```python
from build123d import *

# Parameters (mm, degrees)
SKETCH_1_R          = 32.5
SKETCH_1_R_2        = 17.5
SKETCH_1_R_3        = 2.5
EXTRUDE_1_DEPTH     = 24
SKETCH_2_R          = 35
SKETCH_2_R_2        = 21.5
CUT_EXTRUDE_2_DEPTH = 9
CUT_EXTRUDE_START   = -9
SKETCH_3_R          = 35
SKETCH_3_R_2        = 21.5
CUT_EXTRUDE_3_DEPTH = 9
EXTRUDE_START       = 4
SKETCH_4_R          = 21.5
SKETCH_4_R_2        = 11
EXTRUDE_4_DEPTH     = 4


with BuildPart() as part:
    # Эскиз1 → Вытянуть1 (new body)
    with BuildSketch(Plane.XY):
        Circle(SKETCH_1_R)
        Circle(SKETCH_1_R_2, mode=Mode.SUBTRACT)
        with Locations((-18.438809137, 18.327731563)):
            Circle(SKETCH_1_R_3, mode=Mode.SUBTRACT)
        with Locations((18.327731563, 18.438809137)):
            Circle(SKETCH_1_R_3, mode=Mode.SUBTRACT)
        with Locations((18.438809137, -18.327731563)):
            Circle(SKETCH_1_R_3, mode=Mode.SUBTRACT)
        with Locations((-18.327731563, -18.438809137)):
            Circle(SKETCH_1_R_3, mode=Mode.SUBTRACT)
    extrude(amount=EXTRUDE_1_DEPTH)

    # Эскиз2 → Вытянуть2 (cut)
    with BuildSketch(Plane.XY.offset(24)):
        Circle(SKETCH_2_R)
        Circle(SKETCH_2_R_2, mode=Mode.SUBTRACT)
    extrude(amount=-CUT_EXTRUDE_2_DEPTH, mode=Mode.SUBTRACT)

    # Эскиз3 → Вытянуть3 (cut)
    with BuildSketch(Plane(origin=(0, 0, 0), x_dir=(-1, 0, 0), z_dir=(0, 0, -1)).offset(CUT_EXTRUDE_START)):
        Circle(SKETCH_3_R)
        with Locations(Location((0, 0, 0), (0, 0, 180))):
            Circle(SKETCH_3_R_2, mode=Mode.SUBTRACT)
    extrude(amount=CUT_EXTRUDE_3_DEPTH, mode=Mode.SUBTRACT)

    # Эскиз4 → Вытянуть4 (add)
    with BuildSketch(Plane.XY.offset(24).offset(EXTRUDE_START)):
        Circle(SKETCH_4_R)
        Circle(SKETCH_4_R_2, mode=Mode.SUBTRACT)
    extrude(amount=-EXTRUDE_4_DEPTH)


solid = part.part
```
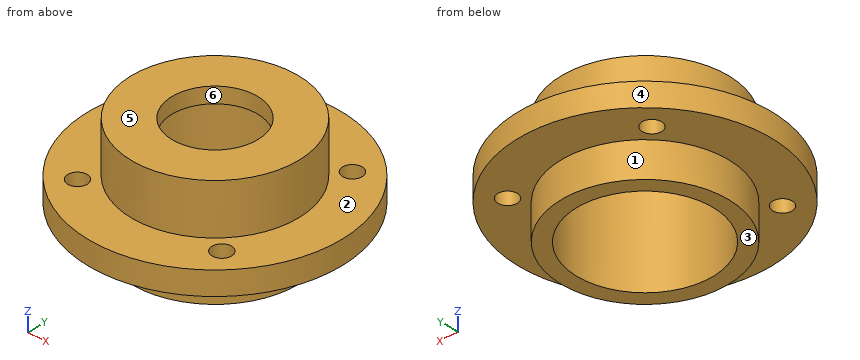
Here's how the part is built. I have some questions about the finished solid (model axes, mm). Face numbers are marked on the shaded views. A direction names the side the tool comes from. Coordinates: 2 decimals unless noted, no trailing zeros. Loops run counter-clockwise (first coordinate to the right, second up) from the corner with the lowest first, then second, coordinate; pieces in that order, holes last. Notation, with made-up numbers: M 45,-30.5 L 98,-30.5 A25 ccw 98,7.5 Z; hole C 41,21.25 d5. An arc over 180 degrees is marked long. One line per item, written item: value.
1. Imagine slicing it at D-D (z = 25). List the corners of the cut face in (x, y) for me.
Geometry says:
outline: C 0,0 d43; hole C 0,0 d22
2. Thinking about a two-plate mould opening in X: for the marked faces 4, 5 and 6, which applies, +X half, -X half, draft (parallel to the pull), parting line (faces both ways), or undercut?
Geometry says:
face 4: parting line
face 5: draft
face 6: undercut
3. Imagine slicing it at A-A (x = 0). List the corners of the cut face in (y, z) for me.
Geometry says:
outline: M -32.5,9 L -21.5,9 L -21.5,0 L -17.5,0 L -17.5,24 L -11,24 L -11,28 L -21.5,28 L -21.5,15 L -32.5,15 Z; M 11,24 L 17.5,24 L 17.5,0 L 21.5,0 L 21.5,9 L 32.5,9 L 32.5,15 L 21.5,15 L 21.5,28 L 11,28 Z
4. Imagine slicing it at C-C (y = -20). List the corners of the cut face in (x, z) for me, and give its area (3 significant figures).
Geometry says:
outline: M -25.62,9 L -20.28,9 L -20.28,15 L -25.62,15 Z; M -16.38,9 L -7.89,9 L -7.89,0 L 7.89,0 L 7.89,9 L 16.58,9 L 16.58,15 L 7.89,15 L 7.89,28 L -7.89,28 L -7.89,15 L -16.38,15 Z; M 20.3,9 L 25.62,9 L 25.62,15 L 20.3,15 Z
area: 609 mm2
5. On a 3-axis mill with a long thin cutter (end or side, diameter ignored), from which of +Z, -Z, +X, -X, +Y, -Y can I reach the whole of each face in a straight line? I mean the marked faces 1, 2 and 3. Say none if no direction works.
Geometry says:
face 1: -Z
face 2: +Z
face 3: -Z, +X, -X, +Y, -Y
6. Please list where these lines run through material, in increasing order: probe 1 along Y at (x, z) = (0, 25.85); probe 2 along X at (y, z) = (-0.5, 3.5); probe 3 along Z at (x, y) = (-10.5, 29.5).
Geometry says:
probe 1: y = -21.5 to -11, 11 to 21.5
probe 2: x = -21.49 to -17.49, 17.49 to 21.49
probe 3: z = 9 to 15
7. Will these pins go through, and if not, where does the flat tip stop? pin 1 Ø4.5 at (x, y) = (18.33, 18.44) entering from +Z; pin 2 Ø1 at (x, z) = (-12, 22) entering from -Y; pin 3 Ø12 at (y, z) = (-8, 13.5) entering from +X; pin 4 Ø8 at (y, z) = (-15, 12.5) entering from -X.
Geometry says:
pin 1: passes through
pin 2: stops at y = -18.17
pin 3: stops at x = 32.44
pin 4: stops at x = -30.58
